Source: CAD feature listing. Evaluate the final solid. Frame: model axes, mm. A direction names the side the tool comes from. Round coordinates to 2 decimals unless told otherwise and drop trailing zeros. Loops run counter-clockwise (first coordinate to the right, second up) from the corner with the lowest first, then second, coordinate; pieces in that order, holes last. Notation, with made-up numbers: (13, 63) -> (56, 63) arc R20 ccw to (56, 95) -> close; hole circle Ø4 at (-24, 86.25). An arc over 180 degrees is marked (long way). Write item = value, one per line.
from build123d import *

# Parameters (mm, degrees)
SKETCH1_W           = 360
SKETCH1_H           = 360
SKETCH1_R           = 15
BOSS_EXTRUDE1_DEPTH = 50
FILLET1_R           = 20
SKETCH2_R           = 105
CUT_EXTRUDE1_DEPTH  = 50
SKETCH3_R           = 23.859856378
CUT_EXTRUDE2_DEPTH  = 10
SKETCH5_R           = 145
SKETCH5_R_2         = 105
SKETCH9_W           = 360
SKETCH9_H           = 360
BOSS_EXTRUDE2_DEPTH = 50
FILLET2_R           = 20
SKETCH10_R          = 105
SKETCH10_R_2        = 15
CUT_EXTRUDE3_DEPTH  = 50
SKETCH11_R          = 30
CUT_EXTRUDE4_DEPTH  = 10
FILLET3_R           = 10


with BuildPart() as part:
    # Sketch1 → Boss-Extrude1 (new body)
    with BuildSketch(Plane(origin=(0, 0, 0), x_dir=(1, 0, 0), z_dir=(0, 1, 0))):
        Rectangle(SKETCH1_W, SKETCH1_H)
        with Locations(Location((-130, 130, 0), (0, 0, 270))):
            Circle(SKETCH1_R, mode=Mode.SUBTRACT)
        with Locations(Location((130, 130, 0), (0, 0, 270))):
            Circle(SKETCH1_R, mode=Mode.SUBTRACT)
        with Locations(Location((130, -130, 0), (0, 0, 270))):
            Circle(SKETCH1_R, mode=Mode.SUBTRACT)
        with Locations(Location((-130, -130, 0), (0, 0, 270))):
            Circle(SKETCH1_R, mode=Mode.SUBTRACT)
    extrude(amount=BOSS_EXTRUDE1_DEPTH)

    # Fillet1
    fillet1_edges = [part.edges().sort_by_distance(p)[0] for p in [
        (-180, 25, -180),
        (180, 25, -180),
        (180, 25, 180),
        (-180, 25, 180),
    ]]
    fillet(fillet1_edges, radius=FILLET1_R)

    # Sketch2 → Cut-Extrude1 (cut)
    with BuildSketch(Plane(origin=(0, 50, 0), x_dir=(1, 0, 0), z_dir=(0, 1, 0))):
        with Locations(Location((0, 0, 0), (0, 0, 270))):
            Circle(SKETCH2_R)
    extrude(amount=-CUT_EXTRUDE1_DEPTH, mode=Mode.SUBTRACT)

    # Sketch3 → Cut-Extrude2 (cut)
    with BuildSketch(Plane(origin=(0, 50, 0), x_dir=(1, 0, 0), z_dir=(0, 1, 0))):
        with Locations(Location((-130, 130, 0), (0, 0, 270))):
            Circle(SKETCH3_R)
        with Locations(Location((130, 130, 0), (0, 0, 270))):
            Circle(SKETCH3_R)
        with Locations(Location((130, -130, 0), (0, 0, 270))):
            Circle(SKETCH3_R)
        with Locations(Location((-130, -130, 0), (0, 0, 270))):
            Circle(SKETCH3_R)
    extrude(amount=-CUT_EXTRUDE2_DEPTH, mode=Mode.SUBTRACT)

    # Sweep-Thin1: sweep along a path in Sketch4
    with BuildLine(Plane.XY) as sweep_thin1_path:
        Line((0, 50), (0, -100))
        ThreePointArc((0, -100), (76.152236891, -283.847763109), (260, -360))
        Line((260, -360), (410, -360))
    # Sketch5 → Sweep-Thin1 (sweep)
    with BuildSketch(Plane(origin=(0, 0, 0), x_dir=(1, 0, 0), z_dir=(0, 1, 0))):
        Circle(SKETCH5_R)
        Circle(SKETCH5_R_2, mode=Mode.SUBTRACT)
    sweep(path=sweep_thin1_path.line)

    # Sketch9 → Boss-Extrude2 (add)
    with BuildSketch(Plane(origin=(410, 0, 0), x_dir=(0, 0, -1), z_dir=(1, 0, 0))):
        with Locations((0, -360)):
            Rectangle(SKETCH9_W, SKETCH9_H)
    extrude(amount=-BOSS_EXTRUDE2_DEPTH)

    # Fillet2
    fillet2_edges = [part.edges().sort_by_distance(p)[0] for p in [
        (385, -540, 180),
        (385, -180, 180),
        (385, -180, -180),
        (385, -540, -180),
    ]]
    fillet(fillet2_edges, radius=FILLET2_R)

    # Sketch10 → Cut-Extrude3 (cut)
    with BuildSketch(Plane(origin=(410, 0, 0), x_dir=(0, 0, -1), z_dir=(1, 0, 0))):
        with Locations(Location((0, -360, 0), (0, 0, 90))):
            Circle(SKETCH10_R)
        with Locations(Location((-130, -230, 0), (0, 0, 90))):
            Circle(SKETCH10_R_2)
        with Locations(Location((130, -230, 0), (0, 0, 90))):
            Circle(SKETCH10_R_2)
        with Locations(Location((130, -490, 0), (0, 0, 90))):
            Circle(SKETCH10_R_2)
        with Locations(Location((-130, -490, 0), (0, 0, 90))):
            Circle(SKETCH10_R_2)
    extrude(amount=-CUT_EXTRUDE3_DEPTH, mode=Mode.SUBTRACT)

    # Sketch11 → Cut-Extrude4 (cut)
    with BuildSketch(Plane(origin=(410, 0, 0), x_dir=(0, 0, -1), z_dir=(1, 0, 0))):
        with Locations(Location((-130, -230, 0), (0, 0, 90))):
            Circle(SKETCH11_R)
        with Locations(Location((130, -230, 0), (0, 0, 90))):
            Circle(SKETCH11_R)
        with Locations(Location((130, -490, 0), (0, 0, 90))):
            Circle(SKETCH11_R)
        with Locations(Location((-130, -490, 0), (0, 0, 90))):
            Circle(SKETCH11_R)
    extrude(amount=-CUT_EXTRUDE4_DEPTH, mode=Mode.SUBTRACT)

    # Fillet3
    fillet3_edges = [part.edges().sort_by_distance(p)[0] for p in [
        (410, -465, 0),
        (0, 50, -105),
    ]]
    fillet(fillet3_edges, radius=FILLET3_R)


solid = part.part
1. Section query B-B (y = -75.5). Return the cut outline in (x, z).
Evaluation:
outline = circle Ø290 at (0, 0); hole circle Ø210 at (0, 0)
2. Section query C-C (y = -230). Give the number of separate pieces and of enclosed holes in the cut face, then the cut area to 3 significant figures.
Evaluation:
separate_pieces = 3
enclosed_holes = 1
area = 71,600 mm²
3. Section query A-A (z = 0). Return the cut outline in (x, y).
Evaluation:
outline = (-180, 0) -> (-145, 0) -> (-145, -100) arc R405 ccw to (260, -505) -> (360, -505) -> (360, -540) -> (410, -540) -> (410, -475) arc R10 ccw to (400, -465) -> (260, -465) arc R365 cw to (-105, -100) -> (-105, 40) arc R10 ccw to (-115, 50) -> (-180, 50) -> close; (105, -100) arc R155 ccw to (260, -255) -> (400, -255) arc R10 ccw to (410, -245) -> (410, -180) -> (360, -180) -> (360, -215) -> (260, -215) arc R115 cw to (145, -100) -> (145, 0) -> (180, 0) -> (180, 50) -> (115, 50) arc R10 ccw to (105, 40) -> close
4. Set-up query: faces 5 (the face through (405.07, -236.503, -159.287)), 6 (the face through (385, -362, 180)), 7 (the face through (140.138, 19.72, -141.056)). Return all of +Z, -Z, +X, -X, +Y, -Y with unobstructed straight access to the full face (end or side cutting, diameter ignored); none if empty.
Evaluation:
face_5 = +X
face_6 = +Z, +X, -X, +Y, -Y
face_7 = +Y
5. Mould query, pull axis Z, two halves, no side actions, for faces 1 (the face through (380.28, -475.693, 134.506)), 2 (the face through (310.7, -221.696, 43.554)), 3 (the face through (384.65, -186.014, 174.297)), 4 (the face through (405.07, -236.503, 100.713)). Classes: released by +Z, released by -Z, zero draft, split by the parting line, or undercut.
Evaluation:
face_1 = undercut
face_2 = split by the parting line
face_3 = released by +Z
face_4 = undercut
6. Contact query for flat-ended pins moving along their axis: pin 1 Ø3 at (x, z) = (287, 66) entering from -Y; pin 2 Ø1.5 at (y, z) = (-383.5, -111.5) entering from +X; pin 3 Ø12 at (y, z) = (-26, 50) entering from +X. Output: stop coordinate, or through.
Evaluation:
pin_1 = -489.86
pin_2 = 410
pin_3 = 138.16
7. Line query: probe 1 along Z at (x, y) = (380, -490); probe 2 along Z at (x, y) = (0, -68). Output: solid intervals per line, ascending. Write a range as from..to.
Evaluation:
probe_1 = -180..-145, -115..115, 145..180
probe_2 = -145..-105, 105..145
